Job drawing, mm, ordinate dimensions from the low corner. One solid piece. A direction names the side the tool comes from. Give positions to 0.01 mm unless a question says otherwise; leave off trailing zeros. Write each loop counter-clockwise with the first axis right and the second up, starting at its lowest first coordinate (ties: lowest second). Pieces come first, ordered by that corner, then holes. Notation, with made-up numbers: (-36, 16) -> (-5, 16) arc R16 cw to (-5, 46) -> close; hole circle Ø5 at (31.25, 82.5). An arc over 180 degrees is marked (long way). One line per question, with ' | ' between items. Start each with the question number.
(1) Pull direction X, two halves, no side cores. Call the marked faces 6, 7, 8 and 9: released by +X, released by -X, zero draft, split by the parting line, or undercut.
(2) Band-saw the part on C-C, the plane x = 52. Give the cut face in (y, z), and give its area (3 significant figures).
(3) Band-saw the part on A-A, the plane y = 8. Count the separate pieces of the cut face and the enclosed holes in it, and give its area (3 significant figures).
(4) Pin check, flat tips, straight feed: P1, Ø1, axis at x = 16, y = 12, coming from the -Z side; P2, Ø1.5, axis at x = 9.5, y = 12.5, coming from the +Z side; P3, Ø7, axis at y = 13, z = 67.5, coming from the -X side; P4, Ø3, axis at x = 34.5, z = 59, coming from the -Y side. Stop position of each tip, or through.
(5) Band-saw the part on B-B, the plane z = 18. Give the cut face in (x, y).
(6) Tool access for the marked faces 1, 2, 3, 4 and 5: list every direction of +Z, -Z, +X, -X, +Y, -Y with a clear straight run to the whole face (end or side of a thin tool).
(7) Drill centre lines: probe 1 along Z at (x, y) = (35, 18); probe 2 along Z at (x, y) = (35, 6.5); probe 3 along Z at (x, y) = (7, 2.75). Where is each one in solid material? Low to high. Write a range as from..to.
(8) Band-saw the part on D-D, the plane y = 24.5. Give the cut face in (x, z).
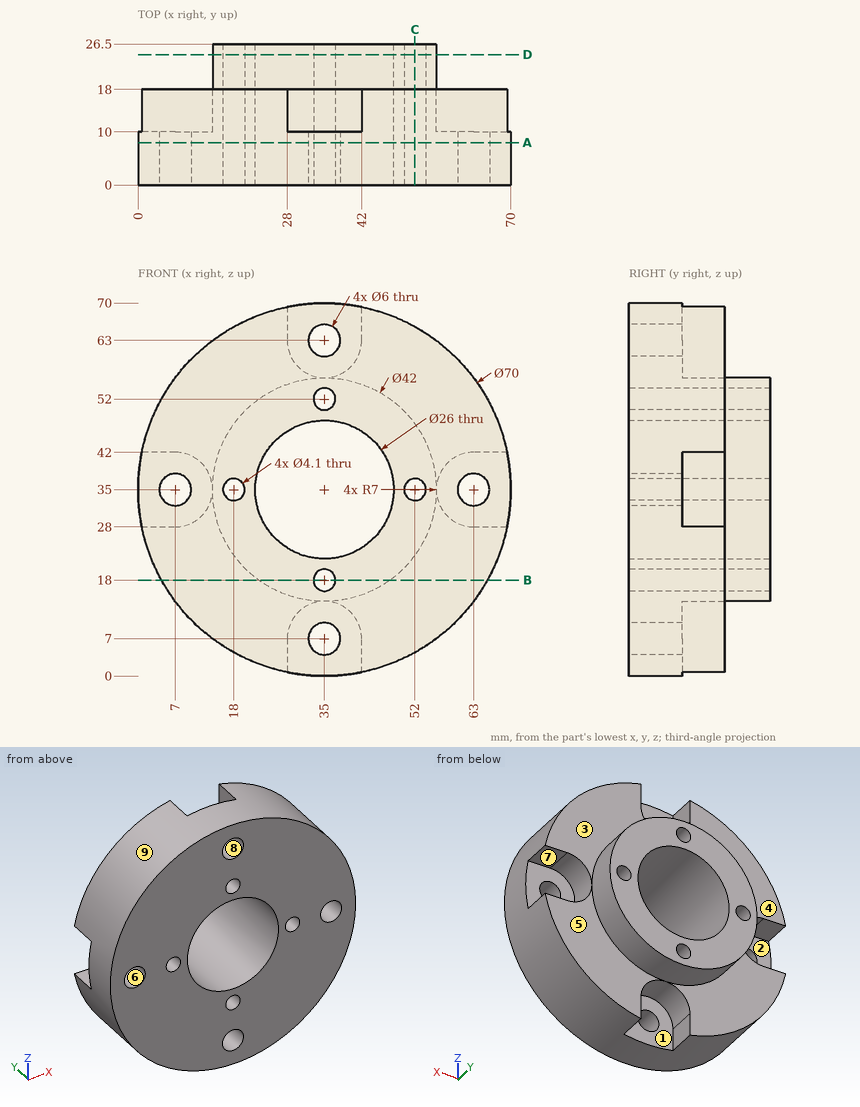
Results:
1) face 6: undercut | face 7: zero draft | face 8: undercut | face 9: split by the parting line
2) outline: (0, 4.41) -> (18, 4.41) -> (18, 22.67) -> (26.5, 22.67) -> (26.5, 32.95) -> (0, 32.95) -> close; (0, 37.05) -> (26.5, 37.05) -> (26.5, 47.33) -> (18, 47.33) -> (18, 65.59) -> (0, 65.59) -> close | area: 1,200 mm²
3) separate pieces: 1 | enclosed holes: 9 | area: 3,150 mm²
4) P1: stops at z = 5.29 | P2: stops at z = 59.75 | P3: stops at x = 15.4 | P4: stops at y = 0
5) outline: (4.41, 0) -> (32.95, 0) -> (32.95, 26.5) -> (22.67, 26.5) -> (22.67, 18) -> (4.41, 18) -> close; (37.05, 0) -> (65.59, 0) -> (65.59, 18) -> (47.33, 18) -> (47.33, 26.5) -> (37.05, 26.5) -> close
6) face 1: -Z, +Y | face 2: -X, +Y | face 3: +Z, +X, +Y | face 4: +Z, -X, +Y | face 5: -Z, +X, +Y
7) probe 1: z = 14..15.95, 20.05..22, 48..49.95, 54.05..56 | probe 2: z = 0..4, 10..15.95, 20.05..22, 48..49.95, 54.05..60, 66..70 | probe 3: z = 14..32, 38..56
8) outline: circle Ø42 at (35, 35); hole circle Ø4.1 at (18, 35); hole circle Ø26 at (35, 35); hole circle Ø4.1 at (35, 18); hole circle Ø4.1 at (35, 52); hole circle Ø4.1 at (52, 35)
